```python
from build123d import *

# Parameters (mm, degrees)
SKETCH11_W         = 69.85
SKETCH11_H         = 22.225
SKETCH11_R         = 3.19405
SKETCH11_R_2       = 4.76885
EXTRUDE3_DEPTH     = 7.9375
CUT_EXTRUDE1_DEPTH = 14.3002
FILLET1_R          = 6.35
EXTRUDE4_DEPTH     = 4.7498
SKETCH15_R         = 13.386908493
CUT_EXTRUDE2_DEPTH = 6.969


with BuildPart() as part:
    # Sketch11 → Extrude3 (new body, symmetric)
    with BuildSketch(Plane.XY):
        with Locations((-28.575, 4.7625)):
            Rectangle(SKETCH11_W, SKETCH11_H)
        Circle(SKETCH11_R, mode=Mode.SUBTRACT)
        with Locations((-28.575, 3.175)):
            Circle(SKETCH11_R_2, mode=Mode.SUBTRACT)
    extrude(amount=EXTRUDE3_DEPTH, both=True)

    # Sketch12 → Cut-Extrude1 (cut)
    with BuildSketch(Plane.XZ.offset(6.35)):
        with BuildLine():
            Line((-7.9248, 4.0894), (6.35, 4.0894))
            Line((6.35, 4.0894), (6.35, -4.0894))
            Line((6.35, -4.0894), (-7.9248, -4.0894))
            ThreePointArc((-7.9248, -4.0894), (-12.0142, 0), (-7.9248, 4.0894))
        make_face()
    extrude(amount=-CUT_EXTRUDE1_DEPTH, mode=Mode.SUBTRACT)

    # Fillet1
    fillet1_edges = [part.edges().sort_by_distance(p)[0] for p in [
        (6.35, -6.35, -6.01345),
        (6.35, 15.875, 0),
        (6.35, -6.35, 6.01345),
    ]]
    fillet(fillet1_edges, radius=FILLET1_R)

    # Sketch13 → Extrude4 (add)
    with BuildSketch(Plane(origin=(0, 15.875, 0), x_dir=(1, 0, 0), z_dir=(0, 1, 0))):
        Polygon((-49.817651581, 0), (-53.483825791, 6.35), (-60.816174209, 6.35), (-64.482348419, 0), (-60.816174209, -6.35), (-53.483825791, -6.35), align=None)
    extrude(amount=EXTRUDE4_DEPTH)

    # Sketch14 → Revolve2 (revolve)
    with BuildSketch(Plane.XY):
        with BuildLine():
            Line((-57.15, 34.183051026), (-60.4139, 36.1442))
            Line((-60.4139, 36.1442), (-61.1124, 35.4457))
            Line((-61.1124, 35.4457), (-61.1124, -8.3058))
            Line((-61.1124, -8.3058), (-70.536908493, -8.3058))
            Line((-70.536908493, -8.3058), (-70.536908493, -9.0678))
            ThreePointArc((-70.536908493, -9.0678), (-64.331959482, -12.927219893), (-57.15, -14.2748))
            Line((-57.15, -14.2748), (-57.15, 34.183051026))
        make_face()
    revolve(axis=Axis((-57.15, 26.585218564, 0), (0, -1, 0)))

    # Sketch15 → Cut-Extrude2 (cut, through all)
    with BuildSketch(Plane(origin=(0, -8.3058, 0), x_dir=(1, 0, 0), z_dir=(0, 1, 0))):
        with Locations((-57.15, 0)):
            Circle(SKETCH15_R)
        Polygon((-57.15, 5.60367982), (-62.75367982, 0), (-57.15, -5.60367982), (-51.54632018, 0), align=None, mode=Mode.SUBTRACT)
    extrude(amount=-CUT_EXTRUDE2_DEPTH, mode=Mode.SUBTRACT)


solid = part.part
```
Build history of the part. All positions in model axes, mm. A direction names the side the tool comes from. Round coordinates to 2 decimals unless told otherwise and drop trailing zeros. Order: outer loops, then holes, each group sorted by start corner. A loop starts at its lowest first (then second) coordinate and runs counter-clockwise, first axis right, second up. Notation, with made-up numbers: (-16, 33) -> (3, 33) arc R25 cw to (3, 71) -> close; hole circle Ø5 at (39, 71.5). An arc over 180 degrees is marked (long way). Answer in a Markdown table with one row per item.
1) Band-saw the part on A-A on x = -1. Give the number of separate pieces and of enclosed holes in the cut face, and give its area (3 significant figures).
Values:
| item | result |
|---|---|
| separate pieces | 3 |
| enclosed holes | 0 |
| area | 189 mm2 |
2) Band-saw the part on D-D on y = 13.5. Give the cut face in (x, z).
Values:
| item | result |
|---|---|
| outline | (-63.5, -7.94) -> (4.95, -7.94) -> (4.95, 7.94) -> (-63.5, 7.94) -> close |
3) Band-saw the part on C-C on y = 24. Give the cut face in (x, z), and give its area (3 significant figures).
Values:
| item | result |
|---|---|
| outline | circle Ø7.92 at (-57.15, 0) |
| area | 49.3 mm2 |
4) Wall check: L1, parallel to X at y = 0, z = 6.8; L2, parallel to X at y = 0.5, z = -6.25; L3, parallel to Y at x = 0, z = -6.5 (3 decimals). Give the ranges that are in metal, low to high.
Values:
| item | result |
|---|---|
| L1 | -63.5 to -32.13, -25.02 to -3.19, 3.19 to 6.35 |
| L2 | -63.5 to -32.52, -24.63 to -3.15, 3.15 to 6.35 |
| L3 | -6.35 to -3.194, 3.194 to 15.875 |
5) Pin check, flat tips, straight feed: P1, Ø5, axis at x = -58.5, y = 19, coming from the +Z side; P2, Ø1.5, axis at y = 26, z = -3, coming from the +X side; P3, Ø2, axis at x = -53, z = 0.5, coming from the +Y side; P4, Ø5, axis at x = -56, y = 25.5, coming from the -Z side. Stop position of each tip, or through.
Values:
| item | result |
|---|---|
| P1 | z = 6.35 |
| P2 | x = -53.89 |
| P3 | y = 36.14 |
| P4 | z = -3.96 |
6) Mould opens along Y. For faces 1 (the cylindrical face through (3.047, 0.959, 5.987)), 2 (the cylindrical face through (4.44, -4.54, -5.99)), 3 (the flat face through (-59.991, -11.051, 2.763)) say: released by +Y, released by -Y, zero draft, split by the parting line, or undercut.
Values:
| item | result |
|---|---|
| face 1 | undercut |
| face 2 | released by -Y |
| face 3 | zero draft |
7) Which spindle directions (+Z, -Z, +X, -X, +Y, -Y) get a long thin tool onto all of the face, cutting with end or side? Do faces 4 (the flat face through (-63.5, 5, 0)), 5 (the cylindrical face through (-60.93, 27.93, -1.19)), 6 (the flat face through (-59.913, -11.051, -2.841)), 7 (the flat face through (-57, 18, 6.35)). Say none if no direction does.
Values:
| item | result |
|---|---|
| face 4 | +Z, -Z, -X, -Y |
| face 5 | +Y |
| face 6 | -Z, -X, -Y |
| face 7 | +Z, +X, -X, +Y |
